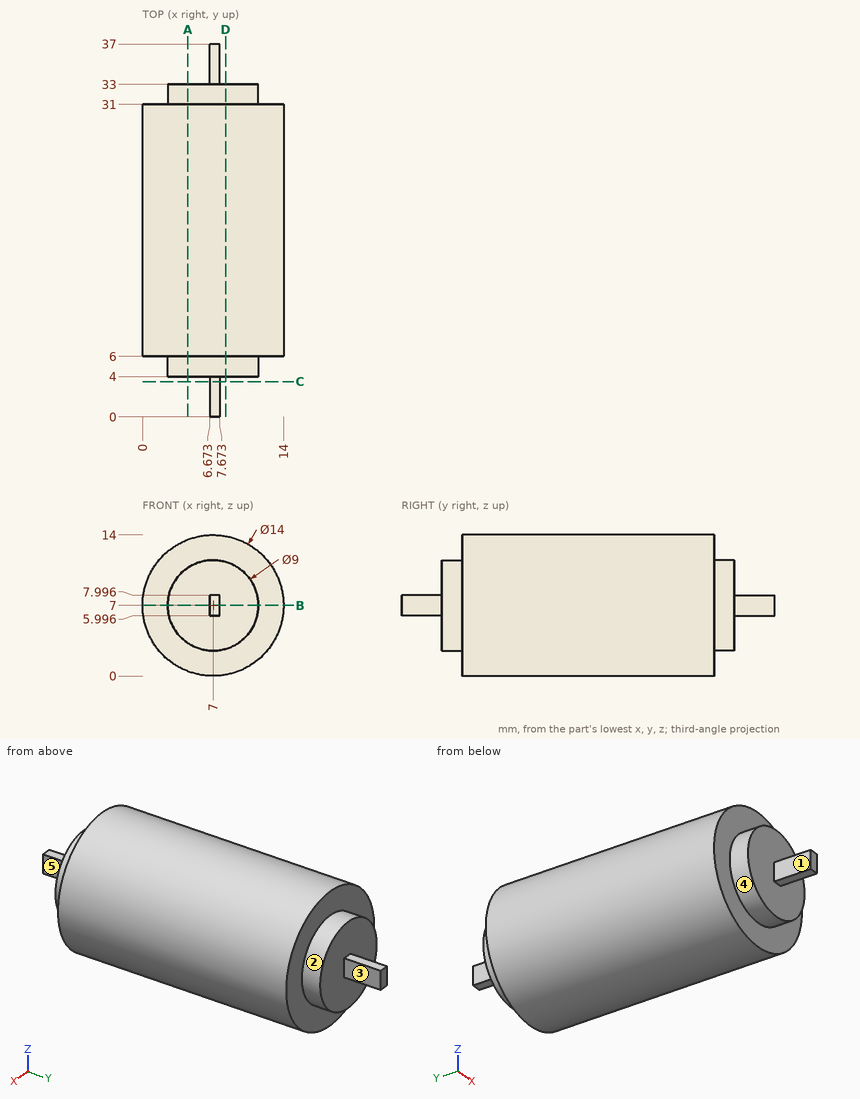
The figure shows three views and two pictorial views of one solid part (mm, origin at its lowest corner). Answer the questions. A direction names the side the tool comes from. Give positions to 0.01 mm unless a question says otherwise; leave off trailing zeros. Order: outer loops, then holes, each group sorted by start corner. A loop starts at its lowest first (then second) coordinate and runs counter-clockwise, first axis right, second up. Notation, with made-up numbers: (80, 11.25) - (126, 11.25) arc R11 ccw to (126, 23.25) - close; hole circle Ø10 at (-17.75, 62). An arc over 180 degrees is marked (long way). Answer as CSV lines item,"result".
Q1. A cutting plane is placed at B-B, the plane z = 7. Determine the outline of the cut face in (x, y).
Answer key:
outline,"(0, 6) - (2.5, 6) - (2.5, 4) - (6.67, 4) - (6.67, 0) - (7.67, 0) - (7.67, 4) - (11.5, 4) - (11.5, 6) - (14, 6) - (14, 31) - (11.5, 31) - (11.5, 33) - (7.67, 33) - (7.67, 37) - (6.67, 37) - (6.67, 33) - (2.5, 33) - (2.5, 31) - (0, 31) - close"
Q2. Straight lines are drawn through the part: L1, parallel to Y at x = 10, z = 6.5; L2, parallel to Y at x = 12.75, z = 5; L3, parallel to X at y = 2, z = 6.75. For each, find the intervals that lie inside material, in ascending order.
Answer key:
L1,"y = 4 to 33"
L2,"y = 6 to 31"
L3,"x = 6.67 to 7.67"
Q3. A cutting plane is placed at A-A, the plane x = 4.5. Determine the outline of the cut face in (y, z).
Answer key:
outline,"(4, 3.26) - (6, 3.26) - (6, 0.46) - (31, 0.46) - (31, 3.26) - (33, 3.26) - (33, 10.74) - (31, 10.74) - (31, 13.54) - (6, 13.54) - (6, 10.74) - (4, 10.74) - close"
Q4. Which of the six approach directions +Z, -Z, +X, -X, +Y, -Y give full straight-line access (tool end or side, diameter ignored) to the marked faces 1, 2, 3, 4 and 5?
Answer key:
face 1,"+Z, -Z, -X, -Y"
face 2,"+Y"
face 3,"+Z, -Z, +X, +Y"
face 4,"-Y"
face 5,"+Z, -Z, +X, -Y"
Q5. Each of these flat-tipped pins is pushed along its axis until it touches: pin 1 Ø1 at (x, z) = (9, 8) entering from -Y; pin 2 Ø0.5 at (x, y) = (7, 36) entering from +Z; pin 3 Ø2 at (y, z) = (34.5, 7.5) entering from -X. Where does it stop, or does it pass through?
Answer key:
pin 1,"stops at y = 4"
pin 2,"stops at z = 8"
pin 3,"stops at x = 6.67"
Q6. A cutting plane is placed at D-D, the plane x = 8.25. Determine the outline of the cut face in (y, z), and give its area (3 significant figures).
Answer key:
outline,"(4, 2.68) - (6, 2.68) - (6, 0.11) - (31, 0.11) - (31, 2.68) - (33, 2.68) - (33, 11.32) - (31, 11.32) - (31, 13.89) - (6, 13.89) - (6, 11.32) - (4, 11.32) - close"
area,"379 mm^2"
Q7. A cutting plane is placed at C-C, the plane y = 3.5. Determine the outline of the cut face in (x, z) (1 decimal).
Answer key:
outline,"(6.7, 6) - (7.7, 6) - (7.7, 8) - (6.7, 8) - close"
